from build123d import *

# Parameters (mm, degrees)
F0_W     = 60
F0_H     = 60
F1_DEPTH = 5
F2_R     = 25
F3_DEPTH = 2
F4_R     = 10
F8_DEPTH = 1


with BuildPart() as f1:
    # F0 (on Top) → F1 (new body)
    with BuildSketch(Plane.XY):
        Rectangle(F0_W, F0_H)
    extrude(amount=F1_DEPTH)

    # F2 (on face) → F3 (cut)
    with BuildSketch(Plane.XY.offset(5)):
        Circle(F2_R)
    extrude(amount=-F3_DEPTH, mode=Mode.SUBTRACT)

    # F4
    f4_edges = [f1.edges().sort_by_distance(p)[0] for p in [
        (30, 30, 2.5),
        (-30, 30, 2.5),
        (30, -30, 2.5),
        (-30, -30, 2.5),
    ]]
    fillet(f4_edges, radius=F4_R)

    # F5 (on Front) → F6 (revolve)
    with BuildSketch(Plane.XZ):
        with BuildLine():
            Line((15, 20), (0, 20))
            Line((0, 20), (0, 0))
            ThreePointArc((0, 0), (8.770167, 9.047375), (15, 20))
        make_face()
        with BuildLine():
            Line((21.891709, 30.538945), (0, 30.538945))
            Line((0, 30.538945), (0, 20))
            Line((0, 20), (15, 20))
            ThreePointArc((15, 20), (15.595579, 27.133347), (21.891709, 30.538945))
        make_face()
        with BuildLine():
            Line((7, 78), (0, 78))
            Line((0, 78), (0, 30.538945))
            Line((0, 30.538945), (21.891709, 30.538945))
            ThreePointArc((21.891709, 30.538945), (24.177264, 57.545259), (9, 80))
            Line((9, 80), (7, 80))
            Line((7, 80), (7, 78))
        make_face()
    revolve(axis=Axis((0, 0, 40), (0, 0, -1)))

    # F7 (on Front) → F8 (join, symmetric)
    with BuildSketch(Plane.XZ):
        Polygon((-21.891709, 30.538945), (-15, 20), (0, 20), (0, 30.538945), align=None)
    extrude(amount=F8_DEPTH, both=True)


solid = f1.part
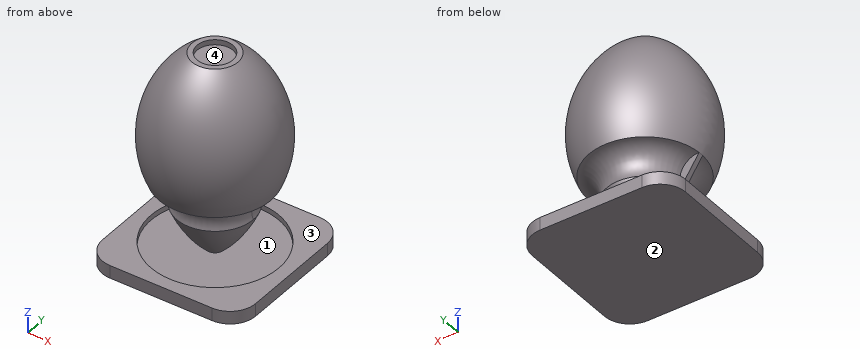
Work out the finished part from the listing and answer in its coordinate system (mm). Face numbers are marked on the shaded views. A direction names the side the tool comes from. Coordinates: 2 decimals unless noted, no trailing zeros. Answer as CSV lines item,"result". Start each with the question number.
Item 1: A tool of negligible diameter and unlimited length cuts with its end or side. For the marked faces 1 and 2, from which of +Z, -Z, +X, -X, +Y, -Y can it reach the whole face along a straight path? Write none if from no direction.
Item 2: Flat-ended cylindrical pins translate along their axes: P1, Ø6, axis at x = -19.5, z = 24, coming from the -Y side; P2, Ø6, axis at x = 3.5, z = 54, coming from the -Y side; P3, Ø10, axis at x = 12, y = 23, coming from the +Z side. Find the tip coordinate at first contact, or state that the pin passes through.
Item 3: Consider L1, parallel to Z at x = -15, y = -23; L2, parallel to X at y = 0, z = 79; L3, parallel to Z at x = 7, y = -9.5. Determine where each line is inside the solid, lowest interval first.
Item 4: Determine the mould class of the marked faces 3 and 4 for opening direction X: released by +X, released by -X, zero draft, split by the parting line, or undercut.
Checks:
1,face 1,"none"
1,face 2,"-Z, +X, -X, +Y, -Y"
2,P1,"stops at y = -1"
2,P2,"stops at y = -25.21"
2,P3,"stops at z = 65.98"
3,L1,"z = 0 to 5"
3,L2,"x = -10.3 to -7, 7 to 10.3"
3,L3,"z = 0 to 3, 13.58 to 77.73"
4,face 3,"zero draft"
4,face 4,"undercut"
